Work out the finished part from the listing and answer in its coordinate system (mm). Face numbers are marked on the shaded views. Coordinates: 2 decimals unless noted, no trailing zeros. Order: outer loops, then holes, each group sorted by start corner. A loop starts at its lowest first (then second) coordinate and runs counter-clockwise, first axis right, second up. Notation, with made-up numbers: M -35.75,61.5 L 9.25,61.5 A19 cw 9.25,68.5 Z; hole C 7,6 d7. An arc over 180 degrees is marked long. Use a Markdown table: item, result.
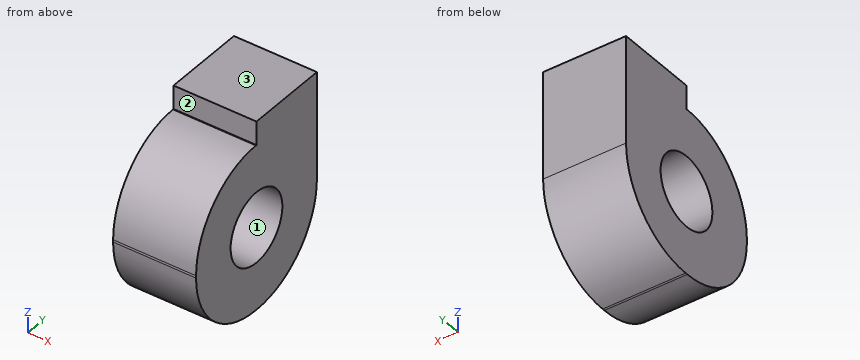
from build123d import *

# Parameters (mm, degrees)
BOX012_W          = 3.5
BOX012_H          = 3.5
BOX012_DEPTH      = 1
CYLINDER003_R     = 1.5
CYLINDER003_DEPTH = 20
BOX011_W          = 3.5
BOX011_H          = 7
BOX011_DEPTH      = 7
FILLET002008002_R = 3.45


with BuildPart() as cube012:
    # Box012 → Box012 (new body)
    with BuildSketch(Plane(origin=(57, 25, 25), x_dir=(1, 0, 0), z_dir=(0, 0, 1))):
        with Locations((1.75, 1.75)):
            Rectangle(BOX012_W, BOX012_H)
    extrude(amount=BOX012_DEPTH)


with BuildPart() as cylinder003:
    # Cylinder003 → Cylinder003 (new body)
    with BuildSketch(Plane(origin=(56, 23, 21.5), x_dir=(0, 0, -1), z_dir=(1, 0, 0))):
        Circle(CYLINDER003_R)
    extrude(amount=CYLINDER003_DEPTH)


with BuildPart() as fusion001:
    # Box011 → Box011 (new body)
    with BuildSketch(Plane(origin=(57, 19.5, 18), x_dir=(1, 0, 0), z_dir=(0, 0, 1))):
        with Locations((1.75, 3.5)):
            Rectangle(BOX011_W, BOX011_H)
    extrude(amount=BOX011_DEPTH)

    # Fillet002008002
    fillet002008002_edges = [fusion001.edges().sort_by_distance(p)[0] for p in [
        (58.75, 19.5, 18),
        (58.75, 19.5, 25),
        (58.75, 26.5, 18),
    ]]
    fillet(fillet002008002_edges, radius=FILLET002008002_R)

    # Cut001: cut Cylinder003
    add(cylinder003.part, mode=Mode.SUBTRACT)


with BuildPart() as fusion001_1:
    # Cut001 placement: moved
    add(fusion001.part.moved(Location((0, 2, 0))))

    # Fusion001: union Cube012
    add(cube012.part)


solid = fusion001_1.part
1. Section C-C on y = 28.25 is taken. Determine the outline of the cut face in (x, z).
Answers below:
| item | result |
|---|---|
| outline | M 57,20.16 L 60.5,20.16 L 60.5,26 L 57,26 Z |
2. For a pull along Z with two mould halves and no side action, classify the marked faces 1, 2 and 3 as +Z half, -Z half, draft (parallel to the pull), parting line (faces both ways), or undercut.
Answers below:
| item | result |
|---|---|
| face 1 | undercut |
| face 2 | draft |
| face 3 | +Z half |
3. Find the intervals of material crossed by probe 1 along Y at (x, z) = (58.5, 21.5); probe 2 along Y at (x, z) = (59.9, 21); probe 3 along Z at (x, y) = (59.7, 25.75), in increasing order.
Answers below:
| item | result |
|---|---|
| probe 1 | 21.5 to 23.5, 26.5 to 28.5 |
| probe 2 | 21.53 to 23.59, 26.41 to 28.47 |
| probe 3 | 18.07 to 20.2, 22.8 to 26 |
4. Section B-B on z = 21 is taken. Determine the outline of the cut face in (x, y), then the cut area to 3 significant figures.
Answers below:
| item | result |
|---|---|
| outline | M 57,21.53 L 60.5,21.53 L 60.5,23.59 L 57,23.59 Z; M 57,26.41 L 60.5,26.41 L 60.5,28.47 L 57,28.47 Z |
| area | 14.4 mm² |
5. Section D-D on z = 24.5 is taken. Determine the outline of the cut face in (x, y).
Answers below:
| item | result |
|---|---|
| outline | M 57,23.16 L 60.5,23.16 L 60.5,28.5 L 57,28.5 Z |
6. Section A-A on x = 57.8 is taken. Determine the outline of the cut face in (y, z), then the cut area to 3 significant figures.
Answers below:
| item | result |
|---|---|
| outline | M 21.5,21.45 A3.45 ccw 24.95,18 L 25.05,18 A3.45 ccw 28.5,21.45 L 28.5,26 L 25,26 L 25,25 L 24.95,25 A3.45 ccw 21.5,21.55 Z; hole C 25,21.5 d3 |
| area | 37.8 mm² |
7. Flat-ended cylindrical pins translate along their axes: P1, Ø1, axis at x = 58, y = 23, coming from the -Z side; P2, Ø2, axis at x = 59, y = 23.5, coming from the -Z side. Find the tip coordinate at first contact, or state that the pin passes through.
Answers below:
| item | result |
|---|---|
| P1 | z = 18.32 |
| P2 | z = 18.03 |
